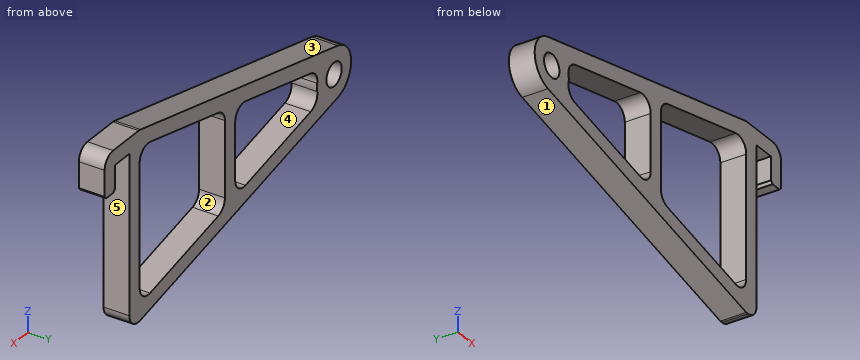
```python
from build123d import *

# Parameters (mm, degrees)
F0_R     = 4.5
F1_DEPTH = 10
F2_R     = 5
F3_SIZE  = 1


with BuildPart() as f1:
    # F0 (on Front) → F1 (new body)
    with BuildSketch(Plane.XZ):
        with BuildLine():
            Line((0, -36), (0, 0))
            Line((0, 0), (0, 30))
            Line((0, 30), (8.5, 30))
            Line((8.5, 30), (8.5, 20))
            Line((8.5, 20), (14.5, 20))
            Line((14.5, 20), (14.5, 36))
            Line((14.5, 36), (8.5, 36))
            Line((8.5, 36), (0, 36))
            Line((0, 36), (-6, 36))
            Line((-6, 36), (-122.203111, 9.754297))
            ThreePointArc((-122.203111, 9.754297), (-130, 0), (-122.203111, -9.754297))
            Line((-122.203111, -9.754297), (-6, -36))
            Line((-6, -36), (0, -36))
        make_face()
        with Locations((-120, 0)):
            Circle(F0_R, mode=Mode.SUBTRACT)
        with BuildLine():
            Line((-111.941284, 5.920903), (-62, 17.200671))
            Line((-62, 17.200671), (-62, -17.200671))
            Line((-62, -17.200671), (-111.941284, -5.920903))
            ThreePointArc((-111.941284, -5.920903), (-110, 0), (-111.941284, 5.920903))
        make_face(mode=Mode.SUBTRACT)
        Polygon((-56, 18.555835), (-6, 29.848864), (-6, -29.848864), (-56, -18.555835), align=None, mode=Mode.SUBTRACT)
    extrude(amount=F1_DEPTH)

    # F2
    f2_edges = [f1.edges().sort_by_distance(p)[0] for p in [
        (-111.941284, -5, -5.920903),
        (-111.941284, -5, 5.920903),
        (-62, -5, -17.200671),
        (-56, -5, 18.555835),
        (-56, -5, -18.555835),
        (-62, -5, 17.200671),
        (-6, -5, 29.848864),
        (-6, -5, -29.848864),
        (14.5, -5, 36),
        (0, -5, -36),
        (-6, -5, 36),
    ]]
    fillet(f2_edges, radius=F2_R)

    # F3
    f3_edges = [f1.edges().sort_by_distance(p)[0] for p in [
        (8.5, -5, 20),
        (14.5, -5, 20),
    ]]
    chamfer(f3_edges, length=F3_SIZE)


solid = f1.part
```
Here's how the part is built. I have some questions about the finished solid (model axes, mm). Face numbers are marked on the shaded views. A direction names the side the tool comes from. Round coordinates to 2 decimals unless told otherwise and drop trailing zeros. Order: outer loops, then holes, each group sorted by start corner. A loop starts at its lowest first (then second) coordinate and runs counter-clockwise, first axis right, second up. Notation, with made-up numbers: (38.25, -34) -> (70.25, -34) arc R8 ccw to (70.25, -30) -> close; hole circle Ø11 at (43.5, 15.25). An arc over 180 degrees is marked (long way). Use a Markdown table: item, result. Add a question column.
(1) Suppose I cut it at A-A, the plane z = 0. Please give me the cut outline in (x, y), and give its area (3 significant figures).
(2) Suppose I cut it at D-D, the plane x = -120. Please give me the cut outline in (y, z), and give its area (3 significant figures).
(3) Suppose I cut it at C-C, the plane x = -90. Please give me the cut outline in (y, z), and give its area (3 significant figures).
(4) For pin 1 Ø2.5 at (x, y) = (5.5, -2.5) entering from -Z; pin 2 Ø8 at (x, z) = (-75.5, -6.5) entering from +Y (1 decimal); pin 3 Ø4.5 at (x, y) = (11.5, -6) entering from -Z; pin 4 Ø6 at (x, y) = (-97.5, -8.5) entering from +Z, each with a flat end and sliding along its axis, tell me the tip position at first contact or that it passes through.
(5) For the marked faces 1 and 2, which set-ups out of +Z, -Z, +X, -X, +Y, -Y let a thin tool reach every point of the face, with its end or its side?
(6) Suppose I cut it at B-B, the plane y = -5.25. Count the separate pieces of the cut face and the enclosed holes in it, and give its area (3 significant figures).
(7) I need wall thicknesses on line 1 along Z through (x, y) = (-78, -9.25); line 2 along Z through (x, y) = (-120, -4.5); line 3 along Z through (x, y) = (-57.5, -5.75). Which ranges of each line are inside material? Lowest first, please.
(8) If we mould it in two halves opening along Z, with no side actions, what happens to the marked faces 3, 4 and 5? For each: released by +Z, released by -Z, zero draft, split by the parting line, or undercut.
Verdict:
| question | item | result |
|---|---|---|
| 1 | outline | (-130, -10) -> (-124.5, -10) -> (-124.5, 0) -> (-130, 0) -> close; (-115.5, -10) -> (-110, -10) -> (-110, 0) -> (-115.5, 0) -> close; (-62, -10) -> (-56, -10) -> (-56, 0) -> (-62, 0) -> close; (-6, -10) -> (0, -10) -> (0, 0) -> (-6, 0) -> close |
| 1 | area | 230 mm2 |
| 2 | outline | (-10, -10.25) -> (0, -10.25) -> (0, -4.5) -> (-10, -4.5) -> close; (-10, 4.5) -> (0, 4.5) -> (0, 10.25) -> (-10, 10.25) -> close |
| 2 | area | 115 mm2 |
| 3 | outline | (-10, -17.03) -> (0, -17.03) -> (0, -10.88) -> (-10, -10.88) -> close; (-10, 10.88) -> (0, 10.88) -> (0, 17.03) -> (-10, 17.03) -> close |
| 3 | area | 123 mm2 |
| 4 | pin 1 | z = 30 |
| 4 | pin 2 | through |
| 4 | pin 3 | z = 20 |
| 4 | pin 4 | z = 16.01 |
| 5 | face 1 | -Z, -X, +Y, -Y |
| 5 | face 2 | +Y, -Y |
| 6 | separate pieces | 1 |
| 6 | enclosed holes | 3 |
| 6 | area | 2,430 mm2 |
| 7 | line 1 | -19.74 to -13.59, 13.59 to 19.74 |
| 7 | line 2 | -10.25 to -4.5, 4.5 to 10.25 |
| 7 | line 3 | -24.37 to 24.37 |
| 8 | face 3 | released by +Z |
| 8 | face 4 | undercut |
| 8 | face 5 | zero draft |
